Drawing for the job (mm, zero at the part's lowest x, y, z). A direction names the side the tool comes from. Coordinates: 2 decimals unless noted, no trailing zeros. Write each loop counter-clockwise with the first axis right and the second up, starting at its lowest first coordinate (ties: lowest second). Pieces come first, ordered by that corner, then holes. Notation, with made-up numbers: M 45.25,-36.75 L 78.25,-36.75 A21 ccw 78.25,0.25 Z; hole C 40.5,43 d4. An arc over 180 degrees is marked long. Use a Markdown table: item, result. Add a question column.
Q1. Wall check: L1, parallel to Y at x = 100, z = 1.05; L2, parallel to X at y = 70, z = 1.5; L3, parallel to Y at x = 100.5, z = 1. Give the ranges that are in metal, low to high. Write a range as from..to.
Q2. Slice it at C-C on z = 9.75. Write the cut outline in (x, y).
Q3. Slice it at B-B on y = 5. Write the cut outline in (x, z).
Q4. Slice it at A-A on x = 5. Write the cut outline in (y, z), then the cut area to 3 significant figures.
Q5. Pin check, flat tips, straight feed: pin 1 Ø3 at (x, z) = (7, 9.5) entering from -Y; pin 2 Ø3 at (x, z) = (99, 10.5) entering from +Y; pin 3 Ø8 at (x, y) = (3, 70.5) entering from +Z. Stop position of each tip, or through.
Q6. Tool access for the marked faces 1, 2 and 3: list every direction of +Z, -Z, +X, -X, +Y, -Y with a clear straight run to the whole face (end or side of a thin tool).
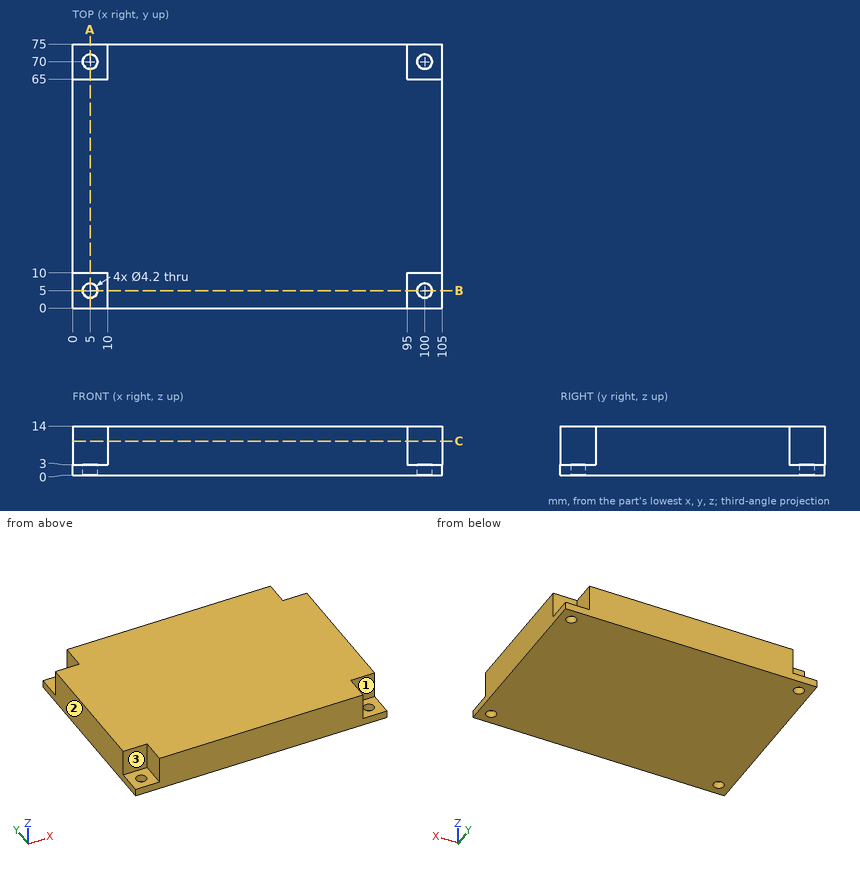
Recorded:
| question | item | result |
|---|---|---|
| 1 | L1 | 0..2.9, 7.1..67.9, 72.1..75 |
| 1 | L2 | 0..2.9, 7.1..97.9, 102.1..105 |
| 1 | L3 | 0..2.96, 7.04..67.96, 72.04..75 |
| 2 | outline | M 0,10 L 10,10 L 10,0 L 95,0 L 95,10 L 105,10 L 105,65 L 95,65 L 95,75 L 10,75 L 10,65 L 0,65 Z |
| 3 | outline | M 0,0 L 2.9,0 L 2.9,3 L 0,3 Z; M 7.1,0 L 97.9,0 L 97.9,3 L 95,3 L 95,14 L 10,14 L 10,3 L 7.1,3 Z; M 102.1,0 L 105,0 L 105,3 L 102.1,3 Z |
| 4 | outline | M 0,0 L 2.9,0 L 2.9,3 L 0,3 Z; M 7.1,0 L 67.9,0 L 67.9,3 L 65,3 L 65,14 L 10,14 L 10,3 L 7.1,3 Z; M 72.1,0 L 75,0 L 75,3 L 72.1,3 Z |
| 4 | area | 805 mm² |
| 5 | pin 1 | y = 10 |
| 5 | pin 2 | y = 65 |
| 5 | pin 3 | z = 3 |
| 6 | face 1 | +Z, +X, -Y |
| 6 | face 2 | +Z, -Z, -X, +Y, -Y |
| 6 | face 3 | +Z, -X, -Y |
